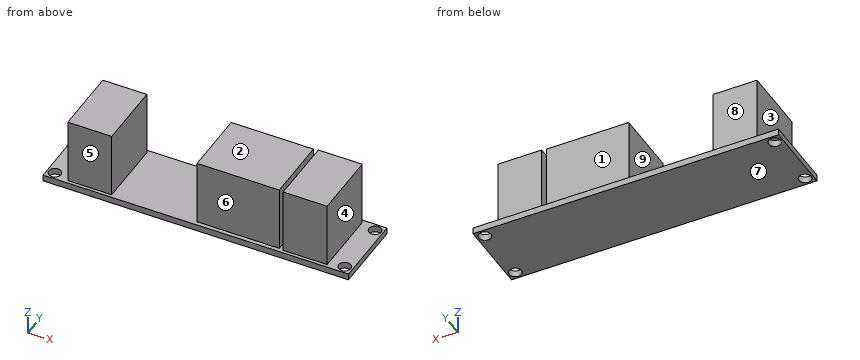
```python
from build123d import *

# Parameters (mm, degrees)
SKETCH_W      = 70.2
SKETCH_H      = 17
SKETCH_R      = 1.4
PAD_DEPTH     = 1.5
SKETCH001_W   = 10.1
SKETCH001_H   = 15.5
SKETCH001_W_2 = 18.9
SKETCH001_H_2 = 15.1
PAD001_DEPTH  = 15.2


with BuildPart() as part:
    # Sketch → Pad (new body)
    with BuildSketch(Plane.XY):
        Rectangle(SKETCH_W, SKETCH_H)
        with Locations((-33.3, 6.7)):
            Circle(SKETCH_R, mode=Mode.SUBTRACT)
        with Locations((33.3, 6.7)):
            Circle(SKETCH_R, mode=Mode.SUBTRACT)
        with Locations((-33.3, -6.7)):
            Circle(SKETCH_R, mode=Mode.SUBTRACT)
        with Locations((33.3, -6.7)):
            Circle(SKETCH_R, mode=Mode.SUBTRACT)
    extrude(amount=PAD_DEPTH)

    # Sketch001 (on Face10 of Pad) → Pad001 (join)
    with BuildSketch(Plane.XY.offset(1.5)):
        with Locations((-24.75, 0)):
            Rectangle(SKETCH001_W, SKETCH001_H)
        with Locations((24.75, 0)):
            Rectangle(SKETCH001_W, SKETCH001_H)
        with Locations((9.25, 0)):
            Rectangle(SKETCH001_W_2, SKETCH001_H_2)
    extrude(amount=PAD001_DEPTH)


solid = part.part
```
Read the model definition and answer for the solid it produces. Units are mm, in the model's axes. Face numbers are marked on the shaded views. A direction names the side the tool comes from. Give positions to 0.01 mm unless a question says otherwise; leave off trailing zeros. Write each loop counter-clockwise with the first axis right and the second up, starting at its lowest first coordinate (ties: lowest second). Pieces come first, ordered by that corner, then holes. Notation, with made-up numbers: M -37,-1 L -13,-1 A13 cw -13,13 Z; hole C 79.25,-39.75 d4. An arc over 180 degrees is marked long. Put each result on its own line as item: value. Start each with the question number.
1. The part is cut by section A-A, the plane x = -33.3. Give the vertices of the cut face in (y, z), and give its area (3 significant figures).
2. Each of these flat-tipped pins is pushed along its axis until it touches: pin 1 Ø2 at (x, z) = (-3, 7.5) entering from -Y; pin 2 Ø3 at (x, z) = (24, 8.5) entering from -Y; pin 3 Ø8 at (x, z) = (-25, 11.5) entering from +Y; pin 4 Ø10 at (y, z) = (-3, 13.5) entering from -X. Where does it stop, or does it pass through?
3. The part is cut by section D-D, the plane x = 5. Give the vertices of the cut face in (y, z).
4. Which of the six approach directions +Z, -Z, +X, -X, +Y, -Y give full straight-line access (tool end or side, diameter ignored) to the marked faces 5, 6, 7, 8 and 9?
5. The part is cut by section C-C, the plane y = -6.7. Give the vertices of the cut face in (x, z).
6. For a pull along X with two mould halves and no side action, classify the marked faces 1, 2, 3 and 4 as released by +X, released by -X, zero draft, split by the parting line, or undercut.
7. Consider line 1 along Y through (x, z) = (-33.3, 0.85); line 2 along X through (y, z) = (0, 6.5); line 3 along Z through (x, y) = (-12, -7). Determine where each line is inside the solid, lowest interval first.
8. The part is cut by section B-B, the plane z = 12.75. Give the vertices of the cut face in (x, y), and give its area (3 significant figures).
Final values:
1. outline: M -8.5,0 L -8.1,0 L -8.1,1.5 L -8.5,1.5 Z; M -5.3,0 L 5.3,0 L 5.3,1.5 L -5.3,1.5 Z; M 8.1,0 L 8.5,0 L 8.5,1.5 L 8.1,1.5 Z
1. area: 17.1 mm²
2. pin 1: passes through
2. pin 2: stops at y = -7.75
2. pin 3: stops at y = 7.75
2. pin 4: stops at x = -29.8
3. outline: M -8.5,0 L 8.5,0 L 8.5,1.5 L 7.55,1.5 L 7.55,16.7 L -7.55,16.7 L -7.55,1.5 L -8.5,1.5 Z
4. face 5: +Z, +X, -X, -Y
4. face 6: +Z, -Y
4. face 7: -Z, +X, -X, +Y, -Y
4. face 8: +Z, +X, -X, +Y
4. face 9: +Z, +Y, -Y
5. outline: M -35.1,0 L -34.7,0 L -34.7,1.5 L -35.1,1.5 Z; M -31.9,0 L 31.9,0 L 31.9,1.5 L 29.8,1.5 L 29.8,16.7 L 19.7,16.7 L 19.7,1.5 L 18.7,1.5 L 18.7,16.7 L -0.2,16.7 L -0.2,1.5 L -19.7,1.5 L -19.7,16.7 L -29.8,16.7 L -29.8,1.5 L -31.9,1.5 Z; M 34.7,0 L 35.1,0 L 35.1,1.5 L 34.7,1.5 Z
6. face 1: undercut
6. face 2: zero draft
6. face 3: released by -X
6. face 4: released by +X
7. line 1: y = -8.5 to -8.1, -5.3 to 5.3, 8.1 to 8.5
7. line 2: x = -29.8 to -19.7, -0.2 to 18.7, 19.7 to 29.8
7. line 3: z = 0 to 1.5
8. outline: M -29.8,-7.75 L -19.7,-7.75 L -19.7,7.75 L -29.8,7.75 Z; M -0.2,-7.55 L 18.7,-7.55 L 18.7,7.55 L -0.2,7.55 Z; M 19.7,-7.75 L 29.8,-7.75 L 29.8,7.75 L 19.7,7.75 Z
8. area: 598 mm²
